Part model, mm, in its own coordinate system. A direction names the side the tool comes from. Round coordinates to 2 decimals unless told otherwise and drop trailing zeros. Loops run counter-clockwise (first coordinate to the right, second up) from the corner with the lowest first, then second, coordinate; pieces in that order, holes last. Notation, with made-up numbers: M 2.25,-32.75 L 7.25,-32.75 A17 cw 7.25,-13.75 Z; hole C -36,20 d10. An arc over 180 degrees is marked long. Put each result on its own line as item: value. Start each with the question number.
1) Slice it at B-B on x = -1. Give the cut face in (y, z).
2) Which spindle directions (+Z, -Z, +X, -X, +Y, -Y) get a long thin tool onto all of the face, cutting with end or side? Do faces 5 (the flat face through (0, 17.5, 5)), 6 (the flat face through (-9, 0, 9)), 7 (the flat face through (7.5, 35, 4)), 8 (the flat face through (7.946, 3.705, 8.085)). Say none if no direction does.
3) Slice it at A-A on y = 31.5. Give the cut face in (x, z).
4) Slice it at D-D on x = -13.5. Give the cut face in (y, z), then the cut area to 3 significant figures.
5) Probe line 1 along Y through (x, z) = (0, 0.6); line 2 along Z through (x, y) = (10.6, 23.75); line 3 along X through (y, z) = (26, 8.5). List the from-to ranges inside material, lowest first.
6) Drop flat-ended pins along their axis: pin 1 Ø6 at (x, y) = (-13.5, 55) entering from -Z; pin 2 Ø6 at (x, y) = (-4, 0) entering from +Z; pin 3 Ø2 at (x, z) = (14, 10) entering from -Y. Give the stop position or say it passes through.
7) Pull direction Y, two halves, no side cores. Call faces 1 (the flat face through (0, 11, 0)), 2 (the flat face through (-8.732, 22.37, 7.936)), 3 (the cylindrical face through (18, 41, 9)), 4 (the cylindrical face through (1.09, 8.51, 9.7)): +Y half, -Y half, draft (parallel to the pull), parting line (faces both ways), or undercut.
8) Slice it at C-C on y = 53.5. Give the cut face in (x, z).
```python
from build123d import *

# Parameters (mm, degrees)
SKETCH1_R           = 12.5
BOSS_EXTRUDE1_DEPTH = 10
SKETCH2_R           = 12.5
SKETCH2_R_2         = 5
BOSS_EXTRUDE2_DEPTH = 1.5
CUT_EXTRUDE3_START  = -3
SKETCH3_R           = 12.5
CUT_EXTRUDE3_DEPTH  = 3
SKETCH4_R           = 12.5
SKETCH4_R_2         = 7.5
BOSS_EXTRUDE3_DEPTH = 4
CUT_EXTRUDE4_START  = -4
SKETCH5_R           = 10
SKETCH5_R_2         = 7.5
CUT_EXTRUDE4_DEPTH  = 4
BOSS_EXTRUDE4_DEPTH = 4
BOSS_EXTRUDE5_START = -1.8
BOSS_EXTRUDE5_DEPTH = 1.8
FILLET1_R           = 3
BOSS_EXTRUDE6_START = -11
BOSS_EXTRUDE6_DEPTH = 11
CUT_EXTRUDE5_DEPTH  = 12.5
CUT_EXTRUDE6_DEPTH  = 2.5
CUT_EXTRUDE7_DEPTH  = 40.080046087
SKETCH12_R          = 2
CUT_EXTRUDE8_DEPTH  = 38.696153679
CUT_EXTRUDE9_DEPTH  = 2.5
FILLET2_R           = 3
SKETCH14_W          = 5
SKETCH14_H          = 11
BOSS_EXTRUDE7_DEPTH = 20
SKETCH15_W          = 15
SKETCH15_H          = 15
BOSS_EXTRUDE8_DEPTH = 3
SKETCH16_W          = 7.5
SKETCH16_H          = 5
CUT_EXTRUDE10_DEPTH = 3
FILLET3_R           = 5


with BuildPart() as part:
    # Sketch1 → Boss-Extrude1 (new body)
    with BuildSketch(Plane.XY):
        Circle(SKETCH1_R)
        Polygon((3.464101615, -6), (6.92820323, 0), (3.464101615, 6), (-3.464101615, 6), (-6.92820323, 0), (-3.464101615, -6), align=None, mode=Mode.SUBTRACT)
    extrude(amount=BOSS_EXTRUDE1_DEPTH)

    # Sketch2 → Boss-Extrude2 (add)
    with BuildSketch(Plane(origin=(0, 0, 0), x_dir=(-1, 0, 0), z_dir=(0, 0, -1))):
        with Locations(Location((0, 0, 0), (0, 0, 180))):
            Circle(SKETCH2_R)
        Circle(SKETCH2_R_2, mode=Mode.SUBTRACT)
    extrude(amount=-BOSS_EXTRUDE2_DEPTH)

    # Sketch3 → Cut-Extrude3 (cut)
    with BuildSketch(Plane.XY.offset(10).offset(CUT_EXTRUDE3_START)):
        Circle(SKETCH3_R)
    extrude(amount=CUT_EXTRUDE3_DEPTH, mode=Mode.SUBTRACT)

    # Sketch4 → Boss-Extrude3 (add)
    with BuildSketch(Plane.XY.offset(7)):
        Circle(SKETCH4_R)
        Circle(SKETCH4_R_2, mode=Mode.SUBTRACT)
    extrude(amount=BOSS_EXTRUDE3_DEPTH)

    # Sketch5 → Cut-Extrude4 (cut)
    with BuildSketch(Plane.XY.offset(11).offset(CUT_EXTRUDE4_START)):
        Circle(SKETCH5_R)
        Circle(SKETCH5_R_2, mode=Mode.SUBTRACT)
    extrude(amount=CUT_EXTRUDE4_DEPTH, mode=Mode.SUBTRACT)

    # Sketch6 → Boss-Extrude4 (add)
    with BuildSketch(Plane.XY.offset(7)):
        with BuildLine():
            ThreePointArc((-6.797308403, -3.169636963), (-7.322220053, -1.623297105), (-7.5, 0))
            Line((-7.5, 0), (-10, 0))
            ThreePointArc((-10, 0), (-9.762960071, -2.164396139), (-9.06307787, -4.226182617))
            Line((-9.06307787, -4.226182617), (-6.797308403, -3.169636963))
        make_face()
        with BuildLine():
            ThreePointArc((6.797308403, 3.169636963), (7.322220053, 1.623297105), (7.5, 0))
            Line((7.5, 0), (10, 0))
            ThreePointArc((10, 0), (9.762960071, 2.164396139), (9.06307787, 4.226182617))
            Line((9.06307787, 4.226182617), (6.797308403, 3.169636963))
        make_face()
    extrude(amount=BOSS_EXTRUDE4_DEPTH)

    # Sketch7 → Boss-Extrude5 (add)
    with BuildSketch(Plane.XY.offset(11).offset(BOSS_EXTRUDE5_START)):
        with BuildLine():
            Line((0, 10), (0, 7.5))
            ThreePointArc((0, 7.5), (4.029747063, 6.325435844), (6.797308403, 3.169636963))
            Line((6.797308403, 3.169636963), (9.06307787, 4.226182617))
            ThreePointArc((9.06307787, 4.226182617), (5.372996083, 8.433914458), (0, 10))
        make_face()
        with BuildLine():
            Line((0, -10), (0, -7.5))
            ThreePointArc((0, -7.5), (-4.029747063, -6.325435844), (-6.797308403, -3.169636963))
            Line((-6.797308403, -3.169636963), (-9.06307787, -4.226182617))
            ThreePointArc((-9.06307787, -4.226182617), (-5.372996083, -8.433914458), (0, -10))
        make_face()
    extrude(amount=BOSS_EXTRUDE5_DEPTH)

    # Fillet1
    # the kernel refuses this fillet: 3 mm, written as the material it takes off along each edge
    with BuildSketch(Plane(origin=(0, 16.873863542, 9.2), x_dir=(1, 0, 0), z_dir=(0, -1, 0))) as fillet1_piece_1_section:
        with BuildLine():
            CenterArc((2.749545417, 3), FILLET1_R, 203.578178478, 66.421821522)
            Line((0, 1.8), (0, 0))
            Line((0, 0), (2.749545417, 0))
        make_face()
    fillet1_piece_1 = extrude(amount=16.247727085, mode=Mode.PRIVATE)
    fillet1_piece_1 = fillet1_piece_1 & Plane(origin=(0, 0, 9.68499996), x_dir=(1, 0, 0), z_dir=(0, 0, -1)) * Cylinder(10, 44, mode=Mode.PRIVATE)
    add(fillet1_piece_1, mode=Mode.SUBTRACT)
    with BuildSketch(Plane(origin=(0, -16.873863542, 9.2), x_dir=(-1, 0, 0), z_dir=(0, 1, 0))) as fillet1_piece_2_section:
        with BuildLine():
            CenterArc((2.749545417, 3), FILLET1_R, 203.578178478, 66.421821522)
            Line((0, 1.8), (0, 0))
            Line((0, 0), (2.749545417, 0))
        make_face()
    fillet1_piece_2 = extrude(amount=16.247727085, mode=Mode.PRIVATE)
    fillet1_piece_2 = fillet1_piece_2 & Plane(origin=(0, 0, 9.68499996), x_dir=(1, 0, 0), z_dir=(0, 0, -1)) * Cylinder(10, 44, mode=Mode.PRIVATE)
    add(fillet1_piece_2, mode=Mode.SUBTRACT)

    # Sketch8 → Boss-Extrude6 (add)
    with BuildSketch(Plane.XY.offset(11).offset(BOSS_EXTRUDE6_START)):
        with BuildLine():
            Line((12.5, 0), (12.5, 30))
            Line((12.5, 30), (-12.5, 30))
            Line((-12.5, 30), (-12.5, 0))
            ThreePointArc((-12.5, 0), (0, 12.5), (12.5, 0))
        make_face()
    extrude(amount=BOSS_EXTRUDE6_DEPTH)

    # Sketch9 → Cut-Extrude5 (cut)
    with BuildSketch(Plane(origin=(0, 30, 0), x_dir=(1, 0, 0), z_dir=(0, 1, 0))):
        Polygon((-7.5, 0), (-7.5, -5.5), (-7.5, -11), (7.5, -11), (7.5, -5.5), (7.5, 0), align=None)
    extrude(amount=-CUT_EXTRUDE5_DEPTH, mode=Mode.SUBTRACT)

    # Sketch10 → Cut-Extrude6 (cut)
    with BuildSketch(Plane(origin=(-7.5, 0, 0), x_dir=(0, 0, -1), z_dir=(1, 0, 0))):
        Polygon((-3.883419246, 26.55), (-5.5, 26.55), (-5.5, 20.95), (-3.883419246, 20.95), (-2.266838493, 23.75), align=None)
        Polygon((-5.5, 20.95), (-5.5, 26.55), (-7.116580754, 26.55), (-8.733161507, 23.75), (-7.116580754, 20.95), align=None)
    extrude(amount=-CUT_EXTRUDE6_DEPTH, mode=Mode.SUBTRACT)

    # Sketch11 → Cut-Extrude7 (cut, through all)
    with BuildSketch(Plane(origin=(-10, 0, 0), x_dir=(0, 0, -1), z_dir=(1, 0, 0))):
        with BuildLine():
            ThreePointArc((-3.5, 23.75), (-4.085786438, 25.164213562), (-5.5, 25.75))
            Line((-5.5, 25.75), (-5.5, 21.75))
            ThreePointArc((-5.5, 21.75), (-4.085786438, 22.335786438), (-3.5, 23.75))
        make_face()
        with BuildLine():
            Line((-5.5, 21.75), (-5.5, 25.75))
            ThreePointArc((-5.5, 25.75), (-7.5, 23.75), (-5.5, 21.75))
        make_face()
    extrude(amount=-CUT_EXTRUDE7_DEPTH, mode=Mode.SUBTRACT)

    # Sketch12 → Cut-Extrude8 (cut, through all)
    with BuildSketch(Plane.ZY.offset(-7.5)):
        with Locations(Location((5.5, 23.75, 0), (0, 0, 180))):
            Circle(SKETCH12_R)
    extrude(amount=-CUT_EXTRUDE8_DEPTH, mode=Mode.SUBTRACT)

    # Sketch13 → Cut-Extrude9 (cut)
    with BuildSketch(Plane.ZY.offset(-7.5)):
        Polygon((8.733161507, 23.75), (7.116580754, 26.55), (3.883419246, 26.55), (2.266838493, 23.75), (3.883419246, 20.95), (7.116580754, 20.95), align=None)
    extrude(amount=-CUT_EXTRUDE9_DEPTH, mode=Mode.SUBTRACT)

    # Fillet2
    fillet2_edges = [part.edges().sort_by_distance(p)[0] for p in [
        (-7.5, 17.5, 5.5),
        (7.5, 17.5, 5.5),
    ]]
    fillet(fillet2_edges, radius=FILLET2_R)

    # Sketch14 → Boss-Extrude7 (add)
    with BuildSketch(Plane(origin=(0, 30, 0), x_dir=(1, 0, 0), z_dir=(0, 1, 0))):
        with Locations((10, -5.5)):
            Rectangle(SKETCH14_W, SKETCH14_H)
        with Locations((-10, -5.5)):
            Rectangle(SKETCH14_W, SKETCH14_H)
    extrude(amount=BOSS_EXTRUDE7_DEPTH)

    # Sketch15 → Boss-Extrude8 (add)
    with BuildSketch(Plane.XY.offset(11)):
        with Locations((0, 42.5)):
            Rectangle(SKETCH15_W, SKETCH15_H)
        Polygon((-12.5, 50), (-7.5, 50), (7.5, 50), (12.5, 50), (12.5, 35), (20, 35), (20, 65), (-20, 65), (-20, 35), (-12.5, 35), align=None)
    extrude(amount=-BOSS_EXTRUDE8_DEPTH)

    # Sketch16 → Cut-Extrude10 (cut)
    with BuildSketch(Plane.XY.offset(11)):
        with Locations((16.25, 37.5)):
            Rectangle(SKETCH16_W, SKETCH16_H)
        with Locations((-16.25, 37.5)):
            Rectangle(SKETCH16_W, SKETCH16_H)
    extrude(amount=-CUT_EXTRUDE10_DEPTH, mode=Mode.SUBTRACT)

    # Fillet3
    fillet3_edges = [part.edges().sort_by_distance(p)[0] for p in [
        (-20, 65, 9.5),
        (20, 65, 9.5),
        (20, 40, 9.5),
        (-20, 40, 9.5),
    ]]
    fillet(fillet3_edges, radius=FILLET3_R)


solid = part.part
```
Recorded:
1. outline: M -12.46,0 L -4.9,0 L -4.9,1.5 L -6,1.5 L -6,7 L -9.95,7 L -9.95,9.76 L -7.43,9.76 L -7.43,11 L -12.46,11 Z; M 4.9,0 L 17.5,0 L 17.5,11 L 9.95,11 L 9.95,7 L 6,7 L 6,1.5 L 4.9,1.5 Z; M 35,8 L 65,8 L 65,11 L 35,11 Z
2. face 5: +Z, -Z
2. face 6: +Z
2. face 7: -Z
2. face 8: none
3. outline: M -12.5,0 L -7.5,0 L -7.5,11 L -12.5,11 Z; M 7.5,0 L 12.5,0 L 12.5,11 L 7.5,11 Z
4. outline: M 40,8 L 65,8 L 65,11 L 40,11 Z
4. area: 75.0 mm2
5. line 1: y = -12.5 to -5, 5 to 17.5
5. line 2: z = 0 to 3.5, 7.5 to 11
5. line 3: x = -12.5 to -7.5, 7.5 to 12.5
6. pin 1: stops at z = 8
6. pin 2: stops at z = 7
6. pin 3: stops at y = 40
7. face 1: draft
7. face 2: undercut
7. face 3: -Y half
7. face 4: undercut
8. outline: M -20,8 L 20,8 L 20,11 L -20,11 Z
